```python
from build123d import *

# Parameters (mm, degrees)
BOSS_EXTRUDE1_DEPTH = 5
SKETCH2_W           = 5
SKETCH2_H           = 90
SKETCH2_H_2         = 40
SKETCH2_W_2         = 35
SKETCH2_H_3         = 5
CUT_EXTRUDE1_DEPTH  = 10
CUT_EXTRUDE2_DEPTH  = 10
FILLET1_R           = 1
FILLET2_R           = 10
CUT_EXTRUDE3_DEPTH  = 10


with BuildPart() as part:
    # Sketch1 → Boss-Extrude1 (new body)
    with BuildSketch(Plane.XY):
        Polygon((80, 33.22), (20, 33.22), (20, 600), (80, 600), (80, 570.05), (85, 570.05), (85, 449.95), (80, 449.95), (80, 390.05), (85, 390.05), (85, 269.95), (80, 269.95), (80, 210.05), (85, 210.05), (85, 89.95), (80, 89.95), align=None)
    extrude(amount=BOSS_EXTRUDE1_DEPTH)

    # Sketch2 → Cut-Extrude1 (cut)
    with BuildSketch(Plane.XY.offset(5)):
        Polygon((67, 370.417424305), (62.417424305, 368.417424305), (70.417424305, 350.087121525), (75, 352.087121525), align=None)
        Polygon((73.902811841, 226.418897298), (51.258042728, 139.314279557), (56.097188159, 138.056236829), (78.741957272, 225.16085457), align=None)
        with Locations((52.33914543, 83.217091399)):
            Rectangle(SKETCH2_W, SKETCH2_H)
        with Locations((42.33914543, 119.314279557)):
            Rectangle(SKETCH2_W, SKETCH2_H_2)
        with Locations((42.5, 377.5)):
            Rectangle(SKETCH2_W_2, SKETCH2_H_3)
    extrude(amount=-CUT_EXTRUDE1_DEPTH, mode=Mode.SUBTRACT)

    # Sketch3 → Cut-Extrude2 (cut)
    with BuildSketch(Plane.XY.offset(5)):
        Polygon((20, 395), (65, 600), (1.513631165, 616.08755832), align=None)
        Polygon((45, 33.22), (20, 58.22), (13.452472792, 20.556075169), align=None)
    extrude(amount=-CUT_EXTRUDE2_DEPTH, mode=Mode.SUBTRACT)

    # Fillet1
    fillet1_edges = [part.edges().sort_by_distance(p)[0] for p in [
        (85, 570.05, 2.5),
        (85, 449.95, 2.5),
        (85, 390.05, 2.5),
        (85, 269.95, 2.5),
        (85, 210.05, 2.5),
        (85, 89.95, 2.5),
    ]]
    fillet(fillet1_edges, radius=FILLET1_R)

    # Fillet2
    fillet2_edges = [part.edges().sort_by_distance(p)[0] for p in [
        (20, 395, 2.5),
        (65, 600, 2.5),
        (45, 33.22, 2.5),
        (20, 58.22, 2.5),
    ]]
    fillet(fillet2_edges, radius=FILLET2_R)

    # Sketch4 → Cut-Extrude3 (cut)
    with BuildSketch(Plane.XY.offset(5)):
        Polygon((60.059418786, 577.492907801), (64.943140501, 576.420871327), (60.654994605, 556.885984463), (55.771272889, 557.958020937), align=None)
    extrude(amount=-CUT_EXTRUDE3_DEPTH, mode=Mode.SUBTRACT)


solid = part.part
```
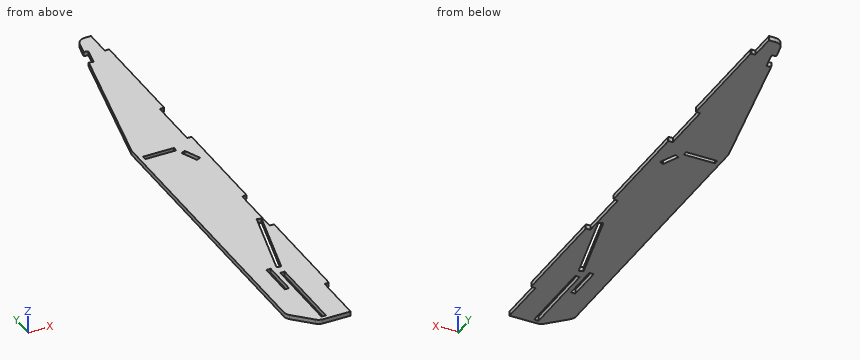
Check sheet for the modelled part. Datum: model origin and axes. Units: mm. Round coordinates to 2 decimals unless told otherwise and drop trailing zeros. Order: outer loops, then holes, each group sorted by start corner. A loop starts at its lowest first (then second) coordinate and runs counter-clockwise, first axis right, second up. Notation, with made-up numbers: (-2.75, 4) -> (56.25, 4) arc R18 cw to (56.25, 39) -> close; hole circle Ø11 at (62, 80). An arc over 180 degrees is marked (long way). One line per item, written item: value. Start each with the question number.
Q1. Cross-section at A-A (y = 194.5). Record the boundary of the cut face in (x, z).
Q2. Cross-section at B-B (x = 34). Record the boundary of the cut face in (y, z), and give its area (3 significant figures).
Q3. Gauge pin test, flat ends, axial feed: pin 1 Ø2 at (x, z) = (82, 2.5) entering from -Y; pin 2 Ø10 at (x, y) = (66.5, 465.5) entering from -Z; pin 3 Ø3 at (x, z) = (66, 1.5) entering from +Y; pin 4 Ø2 at (x, z) = (81.5, 2) entering from +Y. Record the tip position at first contact, or that the pin passes through.
Q4. Thickness scan on line 1 (X direction, y = 115.5, z = 3.75); line 2 (Y direction, x = 82, z = 4.25); line 3 (X direction, y = 244.5, z = 2.9). Record the ranges inside material, lowest first.
Q5. Cross-section at D-D (y = 543.5). Record the boundary of the cut face in (x, z).
Q6. Cross-section at C-C (z = 1.9). Give the number of separate pieces and of enclosed holes in the cut face, and give its area (3 significant figures).
Completed:
1. outline: (20, 0) -> (65.6, 0) -> (65.6, 5) -> (20, 5) -> close; (70.77, 0) -> (85, 0) -> (85, 5) -> (70.77, 5) -> close
2. outline: (44.22, 0) -> (375, 0) -> (375, 5) -> (44.22, 5) -> close; (380, 0) -> (458.78, 0) -> (458.78, 5) -> (380, 5) -> close
2. area: 2,050 mm²
3. pin 1: stops at y = 89.95
3. pin 2: stops at z = 0
3. pin 3: stops at y = 598.32
3. pin 4: stops at y = 570.05
4. line 1: x = 20 to 39.84, 44.84 to 49.84, 54.84 to 85
4. line 2: y = 89.95 to 210.05, 269.95 to 390.05, 449.95 to 570.05
4. line 3: x = 20 to 80
5. outline: (52.6, 0) -> (85, 0) -> (85, 5) -> (52.6, 5) -> close
6. separate pieces: 1
6. enclosed holes: 5
6. area: 29,400 mm²
